```python
from build123d import *

# Parameters (mm, degrees)
BOX011_W               = 0.5
BOX011_H               = 5
BOX011_DEPTH           = 3
BOX011_PLACEMENT_ANGLE = 90
BOX012_W               = 0.5
BOX012_H               = 5
BOX012_DEPTH           = 3
CYLINDER_R             = 1.7
CYLINDER_DEPTH         = 3.9
CYLINDER001_R          = 1.7
CYLINDER001_DEPTH      = 5
BOX010_W               = 6.5
BOX010_H               = 6.5
BOX010_DEPTH           = 4


with BuildPart() as cubo011:
    # Box011 → Box011 (new body)
    with BuildSketch(Plane.XY):
        with Locations((0.25, 2.5)):
            Rectangle(BOX011_W, BOX011_H)
    extrude(amount=BOX011_DEPTH)


with BuildPart() as cubo011_1:
    # Box011 placement: moved
    add(cubo011.part.moved(Location((2.75, -0.25, 3.4))).rotate(Axis((2.75, -0.25, 3.4), (0, 0, 1)), BOX011_PLACEMENT_ANGLE))


with BuildPart() as cubo012:
    # Box012 → Box012 (new body)
    with BuildSketch(Plane(origin=(-0.25, -3, 3.4), x_dir=(1, 0, 0), z_dir=(0, 0, 1))):
        with Locations((0.25, 2.5)):
            Rectangle(BOX012_W, BOX012_H)
    extrude(amount=BOX012_DEPTH)


with BuildPart() as cut004:
    # Cylinder → Cylinder (new body)
    with BuildSketch(Plane.XY):
        Circle(CYLINDER_R)
    extrude(amount=CYLINDER_DEPTH)

    # Cut003: cut Cubo012
    add(cubo012.part, mode=Mode.SUBTRACT)

    # Cut004: cut Cubo011
    add(cubo011_1.part, mode=Mode.SUBTRACT)


with BuildPart() as cilindro001:
    # Cylinder001 → Cylinder001 (new body)
    with BuildSketch(Plane.XY):
        Circle(CYLINDER001_R)
    extrude(amount=CYLINDER001_DEPTH)


with BuildPart() as potentiometer:
    # Box010 → Box010 (new body)
    with BuildSketch(Plane(origin=(-3.25, -3.25, 0), x_dir=(1, 0, 0), z_dir=(0, 0, 1))):
        with Locations((3.25, 3.25)):
            Rectangle(BOX010_W, BOX010_H)
    extrude(amount=BOX010_DEPTH)

    # Cut002: cut Cilindro001
    add(cilindro001.part, mode=Mode.SUBTRACT)

    # Fusion003: union Cut004
    add(cut004.part)


with BuildPart() as potentiometer_1:
    # Fusion003 placement: moved
    add(potentiometer.part.moved(Location((-1, 4.5, 1))))


solid = potentiometer_1.part
```
Verification items for the finished model (mm, model axes). A direction names the side the tool comes from. Coordinates: 2 decimals unless noted, no trailing zeros. Order: outer loops, then holes, each group sorted by start corner. A loop starts at its lowest first (then second) coordinate and runs counter-clockwise, first axis right, second up. Notation, with made-up numbers: (43, -32.75) -> (75, -32.75) arc R29 cw to (75, -11.75) -> close; hole circle Ø7 at (80, -10.5). An arc over 180 degrees is marked (long way). Put each result on its own line as item: value. Start each with the question number.
1) Cross-section at B-B (x = -1). Enter the section's corners in (y, z), plus the area to 3 significant figures.
2) Release check for a two-part mould opening along Y. For faces 1 (the flat face through (-2, 4, 4.9)), 2 (the flat face through (-1, 7.75, 3)), 3 (the flat face through (-2.5, 6, 5)) record: pulls with the +Y half, pulls with the -Y half, needs draft (parallel to the pull), parting line crosses it, or undercut.
3) Cross-section at A-A (y = 4.5). Enter the section's corners in (x, z), plus the area to 3 significant figures.
4) Material ranges on L1, parallel to Y at x = -1, z = 4.5; L2, parallel to X at y = 4.5, z = 4.6; L3, parallel to Z at x = -0.25, y = 5, recorded low to high.
5) Tool access check on faces 4 (the flat face through (0, 4, 4.9)), 5 (the flat face through (2.25, 4, 3)). Record the directions out of +Z, -Z, +X, -X, +Y, -Y that give a thin tool (end or side, any length) a straight path to the whole face; none if there is none.
6) Cross-section at C-C (x = -2.5). Enter the section's corners in (y, z), plus the area to 3 significant figures.
7) Cross-section at D-D (y = 3.5). Enter the section's corners in (x, z).
Geometry check:
1. outline: (1.25, 1) -> (7.75, 1) -> (7.75, 5) -> (6.2, 5) -> (6.2, 4.4) -> (2.8, 4.4) -> (2.8, 5) -> (1.25, 5) -> close
1. area: 24.0 mm^2
2. face 1: undercut
2. face 2: pulls with the +Y half
2. face 3: needs draft
3. outline: (-4.25, 1) -> (2.25, 1) -> (2.25, 5) -> (0.7, 5) -> (0.7, 4.4) -> (-2.7, 4.4) -> (-2.7, 5) -> (-4.25, 5) -> close
3. area: 24.0 mm^2
4. L1: y = 1.25 to 2.8, 6.2 to 7.75
4. L2: x = -4.25 to -2.7, 0.7 to 2.25
4. L3: z = 1 to 4.9
5. face 4: +Z
5. face 5: +Z, -Z, +X, +Y, -Y
6. outline: (1.25, 1) -> (7.75, 1) -> (7.75, 5) -> (5.3, 5) -> (5.3, 4.9) -> (4.75, 4.9) -> (4.75, 4.4) -> (4.25, 4.4) -> (4.25, 4.9) -> (3.7, 4.9) -> (3.7, 5) -> (1.25, 5) -> close
6. area: 25.6 mm^2
7. outline: (-4.25, 1) -> (2.25, 1) -> (2.25, 5) -> (0.37, 5) -> (0.37, 4.9) -> (-0.75, 4.9) -> (-0.75, 4.4) -> (-1.25, 4.4) -> (-1.25, 4.9) -> (-2.37, 4.9) -> (-2.37, 5) -> (-4.25, 5) -> close
